from build123d import *

# Parameters (mm, degrees)
SKETCH1_R           = 35.625
SKETCH1_R_2         = 20
BOSS_EXTRUDE1_DEPTH = 4
SKETCH2_R           = 24
SKETCH2_R_2         = 20
BOSS_EXTRUDE2_DEPTH = 52
FILLET1_R           = 1


with BuildPart() as part:
    # Sketch1 → Boss-Extrude1 (new body)
    with BuildSketch(Plane.XY):
        Circle(SKETCH1_R)
        Circle(SKETCH1_R_2, mode=Mode.SUBTRACT)
    extrude(amount=BOSS_EXTRUDE1_DEPTH)

    # Sketch2 → Boss-Extrude2 (add)
    with BuildSketch(Plane.XY.offset(4)):
        with Locations(Location((0, 0, 0), (0, 0, 180))):
            Circle(SKETCH2_R)
        Circle(SKETCH2_R_2, mode=Mode.SUBTRACT)
    extrude(amount=BOSS_EXTRUDE2_DEPTH)

    # Fillet1
    fillet1_edges = [part.edges().sort_by_distance(p)[0] for p in [
        (24, 0, 4),
    ]]
    fillet(fillet1_edges, radius=FILLET1_R)


solid = part.part
The listing builds one solid part. Answer for the finished solid, in the listing's coordinates (mm). Give positions to 0.01 mm unless a question says otherwise; leave off trailing zeros. Order: outer loops, then holes, each group sorted by start corner. A loop starts at its lowest first (then second) coordinate and runs counter-clockwise, first axis right, second up. Notation, with made-up numbers: (78.5, 38) - (123.5, 38) arc R8 ccw to (123.5, 48) - close; hole circle Ø1 at (-14, 60). An arc over 180 degrees is marked (long way). Answer as CSV lines item,"result".
Q1. A cutting plane is placed at A-A, the plane y = 0. Determine the outline of the cut face in (x, z) (3 decimals), and give its area (3 significant figures).
Answer key:
outline,"(-35.625, 0) - (-20, 0) - (-20, 56) - (-24, 56) - (-24, 5) arc R1 cw to (-25, 4) - (-35.625, 4) - close; (20, 0) - (35.625, 0) - (35.625, 4) - (25, 4) arc R1 cw to (24, 5) - (24, 56) - (20, 56) - close"
area,"541 mm^2"
Q2. Determine the mould class of faces 1 (the face through (7.4, 24.2, 4)), 2 (the face through (-4.336, -19.524, 27.608)), 3 (the face through (-22.89, -7.21, 30.14)) for opening direction Y: pulls with the +Y half, pulls with the -Y half, needs draft (parallel to the pull), parting line crosses it, or undercut.
Answer key:
face 1,"needs draft"
face 2,"undercut"
face 3,"parting line crosses it"
Q3. Each of these flat-tipped pins is pushed along its axis until it touches: pin 1 Ø2 at (y, z) = (25.5, 32) entering from +X; pin 2 Ø2 at (x, y) = (20.5, 21.5) entering from +Z; pin 3 Ø1 at (x, z) = (-4, 47) entering from -Y; pin 4 Ø8 at (y, z) = (1, 18) entering from +X. Where does it stop, or does it pass through?
Answer key:
pin 1,"passes through"
pin 2,"stops at z = 4"
pin 3,"stops at y = -23.74"
pin 4,"stops at x = 24"
Q4. A cutting plane is placed at C-C, the plane z = 17.5. Determine the outline of the cut face in (x, y), and give its area (3 significant figures).
Answer key:
outline,"circle Ø48 at (0, 0); hole circle Ø40 at (0, 0)"
area,"553 mm^2"
Q5. Straight lines are drawn through the part: L1, parallel to Y at x = 0, z = 33; L2, parallel to Y at x = 8.5, z = 24.5. For each, find the intervals that lie inside material, in ascending order.
Answer key:
L1,"y = -24 to -20, 20 to 24"
L2,"y = -22.44 to -18.1, 18.1 to 22.44"
